Could you check a few things on this model? Use its own coordinates, in mm. Give positions to 0.01 mm unless a question says otherwise; leave off trailing zeros.
(1) Imagine slicing it at A-A, the plane z = 1.15. State how many separate pieces and enclosed holes the cut face has, then the cut area to 3 significant figures.
(2) If I drill on probe 1 along X at (y, z) = (37, 0.6); probe 2 along X at (y, z) = (60, 0.7); probe 3 along X at (y, z) = (33.5, 0.6), over which ranges is the centre line in solid material (lowest first)?
(3) Will this pin go through, and if not, where does the flat tip stop? pin 1 (0.8 mm diameter, centred on x = 188.5, z = 0.5, fed in from +Y).
Autodesk Inventor part; units mm, degrees
ref_plane "YZ Plane" through (0, 0, 0) normal (1, 0, 0) x (0, 1, 0)
ref_plane "XZ Plane" through (0, 0, 0) normal (0, 1, 0) x (-1, 0, 0)
ref_plane "XY Plane" through (0, 0, 0) normal (0, 0, 1) x (1, 0, 0)
sketch "スケッチ1" plane through (0, 0, 0) normal (0, 0, 1) x (1, 0, 0)
  line L0 (0, 0) -> (200, 0)
  line L1 (200, 0) -> (200, 100)
  line L2 (200, 100) -> (0, 100)
  line L3 (0, 100) -> (0, 0)
  dimension "d2" = 200
  dimension "d3" = 100
extrude "押し出し1" add sketch "スケッチ1" along normal blind 1.5
fillet "フィレット1" radius 10 2 edges at (0, 100, 0.75) (200, 100, 0.75)
fillet "フィレット2" radius 14 2 edges at (200, 0, 0.75) (0, 0, 0.75)
sketch "スケッチ2" plane through (0, 0, 0) normal (0, 0, -1) x (-1, 0, 0)
  line L0 (-190, 100) -> (-10, 100)
  line L1 (-180, 100) -> (-20, 100)
  line L2 (-20, 100) -> (-20, 116)
  line L3 (-20, 116) -> (-180, 116)
  line L4 (-180, 116) -> (-180, 100)
  line L5 (0, 90) -> (0, 14)
  line L6 (-200, 14) -> (-200, 90)
  point P0 (0, 0)
  dimension "d6" = 20
  dimension "d7" = 20
  dimension "d8" = 16
extrude "押し出し2" add sketch "スケッチ2" against normal blind 1.5
fillet "フィレット3" radius 6 4 edges at (20, 100, 0.75) (20, 116, 0.75) (180, 116, 0.75) (180, 100, 0.75)
sketch "スケッチ3" plane through (0, 0, 0) normal (0, 0, -1) x (-1, 0, 0)
  line L0 (-14, 0) -> (-186, 0)
  line L1 (-200, 14) -> (-200, 90)
  line L2 (0, 90) -> (0, 14)
  point P0 (0, 0)
  point P1 (-167, 7)
  point P2 (-167, 37)
  point P3 (-191, 37)
  point P4 (-191, 7)
  point P5 (-9, 7)
  point P6 (-33, 7)
  point P7 (-9, 37)
  point P8 (-33, 37)
  dimension "d12" = 7
  dimension "d13" = 7
  dimension "d14" = 9
  dimension "d15" = 9
  dimension "d16" = 30
  dimension "d17" = 24
  dimension "d18" = 24
  dimension "d19" = 30
  dimension "d27" = 7
  dimension "d28" = 9
  dimension "d31" = 24
  dimension "d34" = 30
hole "穴1" at (167, 7, 0) at (167, 37, 0) at (191, 37, 0) at (191, 7, 0) at (9, 7, 0) at (9, 37, 0) at (33, 37, 0) at (33, 7, 0) direction (0, 0, 1) diameter 3.5 end through all
sketch "スケッチ4" plane through (0, 0, 1.5) normal (0, 0, 1) x (1, 0, 0)
  line L0 (174, 116) -> (26, 116)
  line L1 (85, 116) -> (115, 116)
  line L2 (115, 116) -> (115, 96)
  line L3 (115, 96) -> (85, 96)
  line L4 (85, 96) -> (85, 116)
  line L5 (100, 116) -> (100, 0)
  line L6 (14, 0) -> (186, 0)
  point P0 (0, 0)
  dimension "d37" = 30
  dimension "d38" = 20
extrude "押し出し3" cut sketch "スケッチ4" against normal through all
fillet "フィレット4" radius 2 2 edges at (85, 116, 0.75) (115, 116, 0.75)
sketch "スケッチ5" plane through (0, 0, 1.5) normal (0, 0, 1) x (1, 0, 0)
  circle A0 centre (10, 60) radius 1.5
  circle A1 centre (60, 100) radius 1.5
  circle A2 centre (60, 10) radius 1.5
  circle A3 centre (140, 10) radius 1.5
  circle A4 centre (190, 60) radius 1.5
  circle A5 centre (140, 100) radius 1.5
  point P0 (0, 0)
hole "穴2" at (60, 10, 1.5) at (10, 60, 1.5) at (60, 100, 1.5) at (140, 100, 1.5) at (190, 60, 1.5) at (140, 10, 1.5) direction (0, 0, -1) diameter 3.5 end through all
sketch "スケッチ6" plane through (0, 0, 1.5) normal (0, 0, 1) x (1, 0, 0)
  line L0 (14, 40.66) -> (80.04, 40.66)
  line L1 (14, 94) -> (14, 40.66)
  line L2 (80.04, 94) -> (14, 94)
  line L3 (80.04, 81.046) -> (80.04, 94)
  line L4 (82.58, 78.506) -> (80.04, 81.046)
  line L5 (82.58, 45.74) -> (82.58, 78.506)
  line L6 (80.04, 43.2) -> (82.58, 45.74)
  line L7 (80.04, 40.66) -> (80.04, 43.2)
  circle A0 centre (47.02, 43.2) radius 0.4
  circle A1 centre (49.56, 43.2) radius 0.4
  circle A2 centre (52.1, 43.2) radius 0.4
  circle A3 centre (54.64, 43.2) radius 0.4
  circle A4 centre (57.18, 43.2) radius 0.4
  circle A5 centre (59.72, 43.2) radius 0.4
  circle A6 centre (64.8, 43.2) radius 0.4
  circle A7 centre (67.34, 43.2) radius 0.4
  circle A8 centre (69.88, 43.2) radius 0.4
  circle A9 centre (72.42, 43.2) radius 0.4
  circle A10 centre (74.96, 43.2) radius 0.4
  circle A11 centre (77.5, 43.2) radius 0.4
  circle A12 centre (37.876, 91.46) radius 0.4
  circle A13 centre (40.416, 91.46) radius 0.4
  circle A14 centre (42.956, 91.46) radius 0.4
  circle A15 centre (45.496, 91.46) radius 0.4
  circle A16 centre (48.036, 91.46) radius 0.4
  circle A17 centre (50.576, 91.46) radius 0.4
  circle A18 centre (53.116, 91.46) radius 0.4
  circle A19 centre (55.656, 91.46) radius 0.4
  circle A20 centre (64.8, 91.46) radius 0.4
  circle A21 centre (67.34, 91.46) radius 0.4
  circle A22 centre (69.88, 91.46) radius 0.4
  circle A23 centre (72.42, 91.46) radius 0.4
  circle A24 centre (74.96, 91.46) radius 0.4
  circle A25 centre (77.5, 91.46) radius 0.4
  circle A26 centre (76.865, 53.233) radius 0.4
  circle A27 centre (76.865, 60.853) radius 0.4
  circle A28 centre (74.325, 53.233) radius 0.4
  circle A29 centre (74.325, 60.853) radius 0.4
  circle A30 centre (71.785, 53.233) radius 0.4
  circle A31 centre (71.785, 60.853) radius 0.4
  circle A32 centre (69.245, 53.233) radius 0.4
  circle A33 centre (69.245, 60.853) radius 0.4
  circle A34 centre (66.705, 53.233) radius 0.4
  circle A35 centre (66.705, 60.853) radius 0.4
  circle A36 centre (64.165, 53.233) radius 0.4
  circle A37 centre (64.165, 60.853) radius 0.4
  circle A38 centre (61.625, 53.233) radius 0.4
  circle A39 centre (61.625, 60.853) radius 0.4
  circle A40 centre (59.085, 53.233) radius 0.4
  circle A41 centre (59.085, 60.853) radius 0.4
  circle A42 centre (56.545, 53.233) radius 0.4
  circle A43 centre (56.545, 60.853) radius 0.4
  circle A44 centre (54.005, 53.233) radius 0.4
  circle A45 centre (54.005, 60.853) radius 0.4
  circle A46 centre (51.465, 53.233) radius 0.4
  circle A47 centre (51.465, 60.853) radius 0.4
  circle A48 centre (48.925, 53.233) radius 0.4
  circle A49 centre (48.925, 60.853) radius 0.4
  circle A50 centre (46.385, 53.233) radius 0.4
  circle A51 centre (46.385, 60.853) radius 0.4
  circle A52 centre (43.845, 53.233) radius 0.4
  circle A53 centre (43.845, 60.853) radius 0.4
  circle A54 centre (30.383, 66.822) radius 0.5
  circle A55 centre (35.463, 66.822) radius 0.5
  circle A56 centre (32.288, 80.538) radius 0.4
  circle A57 centre (34.828, 80.538) radius 0.4
  circle A58 centre (34.828, 83.078) radius 0.4
  circle A59 centre (32.288, 83.078) radius 0.4
  circle A60 centre (29.748, 85.618) radius 0.4
  circle A61 centre (32.288, 85.618) radius 0.4
  circle A62 centre (34.828, 85.618) radius 0.4
  circle A63 centre (34.828, 88.158) radius 0.4
  circle A64 centre (32.288, 88.158) radius 0.4
  circle A65 centre (29.748, 88.158) radius 0.4
  circle A66 centre (77.64, 71.09) radius 0.4
  circle A67 centre (77.64, 68.55) radius 0.4
  circle A68 centre (77.64, 66.01) radius 0.4
  circle A69 centre (80.18, 66.01) radius 0.4
  circle A70 centre (80.18, 68.55) radius 0.4
  circle A71 centre (80.18, 71.09) radius 0.4
  circle A72 centre (62.26, 91.46) radius 0.4
  circle A73 centre (35.336, 91.46) radius 0.4
  circle A74 centre (59.72, 91.46) radius 0.4
  circle A75 centre (44.48, 43.2) radius 0.4
  circle A76 centre (32.796, 91.46) radius 0.4
  circle A77 centre (41.94, 43.2) radius 0.4
  circle A78 centre (29.24, 91.46) radius 1.5875
  circle A79 centre (27.97, 43.2) radius 1.5875
  circle A80 centre (80.04, 76.22) radius 1.5875
  circle A81 centre (80.04, 48.28) radius 1.5875
  point P0 (0, 0)
hole "穴3" at (29.24, 91.46, 1.5) at (27.97, 43.2, 1.5) at (80.04, 48.28, 1.5) at (80.04, 76.22, 1.5) direction (0, 0, -1) diameter 3.5 end through all
sketch "スケッチ7" plane through (0, 0, 1.5) normal (0, 0, 1) x (1, 0, 0)
  line L0 (177, 86) -> (98, 86)
  arc A0 (180, 83) -> (177, 86) centre (177, 83) ccw
  line L1 (180, 33) -> (180, 83)
  arc A1 (177, 30) -> (180, 33) centre (177, 33) ccw
  line L2 (98, 30) -> (177, 30)
  arc A2 (95, 33) -> (98, 30) centre (98, 33) ccw
  line L3 (95, 83) -> (95, 33)
  arc A3 (98, 86) -> (95, 83) centre (98, 83) ccw
  circle A4 centre (98.5, 33.5) radius 3
  circle A5 centre (156.5, 33.5) radius 3
  circle A6 centre (157.77, 75.09) radius 0.5
  circle A7 centre (155.23, 75.09) radius 0.5
  circle A8 centre (108.45, 83.77) radius 0.5
  circle A9 centre (110.99, 83.77) radius 0.5
  circle A10 centre (113.53, 83.77) radius 0.5
  circle A11 centre (116.07, 83.77) radius 0.5
  circle A12 centre (118.61, 83.77) radius 0.5
  circle A13 centre (121.15, 83.77) radius 0.5
  circle A14 centre (123.69, 83.77) radius 0.5
  circle A15 centre (126.23, 83.77) radius 0.5
  circle A16 centre (128.77, 83.77) radius 0.5
  circle A17 centre (131.31, 83.77) radius 0.5
  circle A18 centre (133.85, 83.77) radius 0.5
  circle A19 centre (136.39, 83.77) radius 0.5
  circle A20 centre (138.93, 83.77) radius 0.5
  circle A21 centre (141.47, 83.77) radius 0.5
  circle A22 centre (144.01, 83.77) radius 0.5
  circle A23 centre (146.55, 83.77) radius 0.5
  circle A24 centre (149.09, 83.77) radius 0.5
  circle A25 centre (151.63, 83.77) radius 0.5
  circle A26 centre (103.37, 81.23) radius 0.5
  circle A27 centre (105.91, 81.23) radius 0.5
  circle A28 centre (108.45, 81.23) radius 0.5
  circle A29 centre (110.99, 81.23) radius 0.5
  circle A30 centre (113.53, 81.23) radius 0.5
  circle A31 centre (116.07, 81.23) radius 0.5
  circle A32 centre (118.61, 81.23) radius 0.5
  circle A33 centre (121.15, 81.23) radius 0.5
  circle A34 centre (123.69, 81.23) radius 0.5
  circle A35 centre (126.23, 81.23) radius 0.5
  circle A36 centre (128.77, 81.23) radius 0.5
  circle A37 centre (131.31, 81.23) radius 0.5
  circle A38 centre (133.85, 81.23) radius 0.5
  circle A39 centre (136.39, 81.23) radius 0.5
  circle A40 centre (138.93, 81.23) radius 0.5
  circle A41 centre (141.47, 81.23) radius 0.5
  circle A42 centre (144.01, 81.23) radius 0.5
  circle A43 centre (146.55, 81.23) radius 0.5
  circle A44 centre (149.09, 81.23) radius 0.5
  circle A45 centre (151.63, 81.23) radius 0.5
  circle A46 centre (109.5, 50.5) radius 0.5
  circle A47 centre (104.5, 50.5) radius 0.5
  circle A48 centre (107, 50.5) radius 0.5
  circle A49 centre (105.91, 83.77) radius 0.5
  circle A50 centre (103.37, 83.77) radius 0.5
  circle A51 centre (155.23, 77.63) radius 0.5
  circle A52 centre (157.77, 77.63) radius 0.5
  circle A53 centre (156.5, 82.5) radius 3
  circle A54 centre (98.5, 82.5) radius 3
  point P0 (0, 0)
hole "穴4" at (156.5, 33.5, 1.5) at (98.5, 33.5, 1.5) at (98.5, 82.5, 1.5) at (156.5, 82.5, 1.5) direction (0, 0, -1) diameter 3.5 end through all
properties part number "upper_frame" material "アルミニウム 6061"
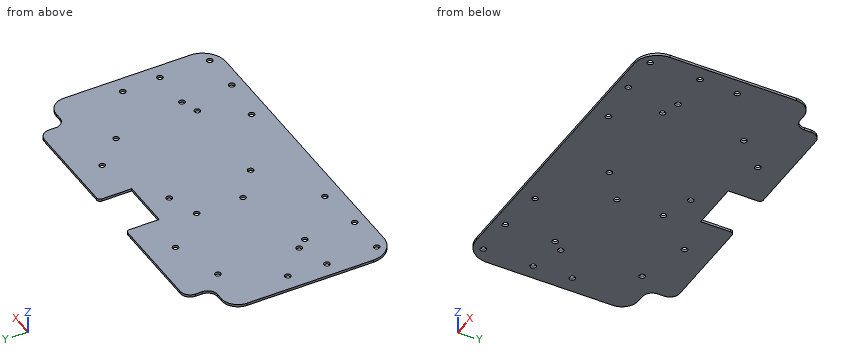
Answer block:
1. separate pieces: 1
1. enclosed holes: 22
1. area: 21,600 mm2
2. probe 1: x = 0 to 7.25, 10.75 to 31.25, 34.75 to 165.25, 168.75 to 189.25, 192.75 to 200
2. probe 2: x = 0 to 8.25, 11.75 to 188.25, 191.75 to 200
2. probe 3: x = 0 to 96.75, 100.25 to 154.75, 158.25 to 200
3. pin 1: stops at y = 100
